Verification items for the finished model (mm, model axes). A direction names the side the tool comes from. Coordinates: 2 decimals unless noted, no trailing zeros. Write each loop counter-clockwise with the first axis right and the second up, starting at its lowest first coordinate (ties: lowest second). Pieces come first, ordered by that corner, then holes.
```python
from build123d import *

# Parameters (mm, degrees)
PAD_DEPTH       = 6.1
SKETCH001_R     = 1.75
POCKET_DEPTH    = 5.001
POCKET001_DEPTH = 3.8
FILLET_R        = 1.5


with BuildPart() as part:
    # Sketch → Pad (new body, symmetric)
    with BuildSketch(Plane.XZ):
        Polygon((-6, 3.7), (-4, 3.7), (-4, 5), (4, 5), (4, 3.7), (6, 3.7), (6, 2.7), (3.6, 0), (-3.6, 0), (-6, 2.7), align=None)
    extrude(amount=PAD_DEPTH, both=True)

    # Sketch001 (on Face4 of Pad) → Pocket (cut, through all)
    with BuildSketch(Plane(origin=(0, 0, 5), x_dir=(-1, 0, 0), z_dir=(0, 0, 1))):
        Circle(SKETCH001_R)
    extrude(amount=-POCKET_DEPTH, mode=Mode.SUBTRACT)

    # Sketch002 (on Face7 of Pocket) → Pocket001 (cut)
    with BuildSketch(Plane(origin=(0, 0, 0), x_dir=(1, 0, 0), z_dir=(0, 0, -1))):
        Polygon((2.9, 1.674316), (0, 3.348632), (-2.9, 1.674316), (-2.9, -1.674316), (0, -3.348632), (2.9, -1.674316), align=None)
    extrude(amount=-POCKET001_DEPTH, mode=Mode.SUBTRACT)

    # Fillet
    fillet_edges = [part.edges().sort_by_distance(p)[0] for p in [
        (3.6, 0, 0),
        (-3.6, 0, 0),
    ]]
    fillet(fillet_edges, radius=FILLET_R)


solid = part.part
```
1. Sectioned sample at A-A, the plane z = 1.35. Record the boundary of the cut face in (x, y).
2. Gauge pin test, flat ends, axial feed: P1, Ø1.6, axis at x = 4.5, y = 2.5, coming from the +Z side; P2, Ø0.6, axis at x = -5, y = -1.5, coming from the +Z side; P3, Ø3, axis at x = 0, y = 0, coming from the -Z side; P4, Ø0.6, axis at y = 2, z = 4.5, coming from the -X side. Record the tip position at first contact, or that the pin passes through.
3. Material ranges on L1, parallel to Y at x = 0, z = 4.25; L2, parallel to X at y = 0, z = 4.5; L3, parallel to X at y = -1.5, z = 3.5, recorded low to high.
4. Sectioned sample at D-D, the plane y = -3.5. Record the boundary of the cut face in (x, z).
5. Tool access check on faces 1 (the flat face through (-1.47, 2.5, 1.87)), 2 (the cylindrical face through (3.549, 0.085, 0.135)), 3 (the flat face through (4, 0, 4)). Record the directions out of +Z, -Z, +X, -X, +Y, -Y that give a thin tool (end or side, any length) a straight path to the whole face; none if there is none.
6. Draft check along Y on faces 4 (the flat face through (1.43, 2.523, 1.873)), 5 (the flat face through (0, 6.1, 3)), 6 (the flat face through (-2, 0, 5)), 7 (the flat face through (-2.9, 0, 2)). Enter one of: pulls with the +Y half, pulls with the -Y half, needs draft (parallel to the pull), parting line crosses it, or undercut.
7. Sectioned sample at C-C, the plane x = 1.25. Record the boundary of the cut face in (y, z).
Outcome:
1. outline: (-4.8, -6.1) - (4.8, -6.1) - (4.8, 6.1) - (-4.8, 6.1) - close; hole (-2.9, -1.67) - (0, -3.35) - (2.9, -1.67) - (2.9, 1.67) - (0, 3.35) - (-2.9, 1.67) - close
2. P1: stops at z = 5
2. P2: stops at z = 3.7
2. P3: passes through
2. P4: stops at x = -4
3. L1: y = -6.1 to -1.75, 1.75 to 6.1
3. L2: x = -4 to -1.75, 1.75 to 4
3. L3: x = -6 to -2.9, 2.9 to 6
4. outline: (-6, 2.7) - (-4.05, 0.5) arc R1.5 ccw to (-2.93, 0) - (2.93, 0) arc R1.5 ccw to (4.05, 0.5) - (6, 2.7) - (6, 3.7) - (4, 3.7) - (4, 5) - (-4, 5) - (-4, 3.7) - (-6, 3.7) - close
5. face 1: -Z
5. face 2: -Z, +X, +Y, -Y
5. face 3: +Z, +X, +Y, -Y
6. face 4: undercut
6. face 5: pulls with the +Y half
6. face 6: needs draft
6. face 7: undercut
7. outline: (-6.1, 0) - (-2.63, 0) - (-2.63, 3.8) - (-1.22, 3.8) - (-1.22, 5) - (-6.1, 5) - close; (1.22, 3.8) - (2.63, 3.8) - (2.63, 0) - (6.1, 0) - (6.1, 5) - (1.22, 5) - close
